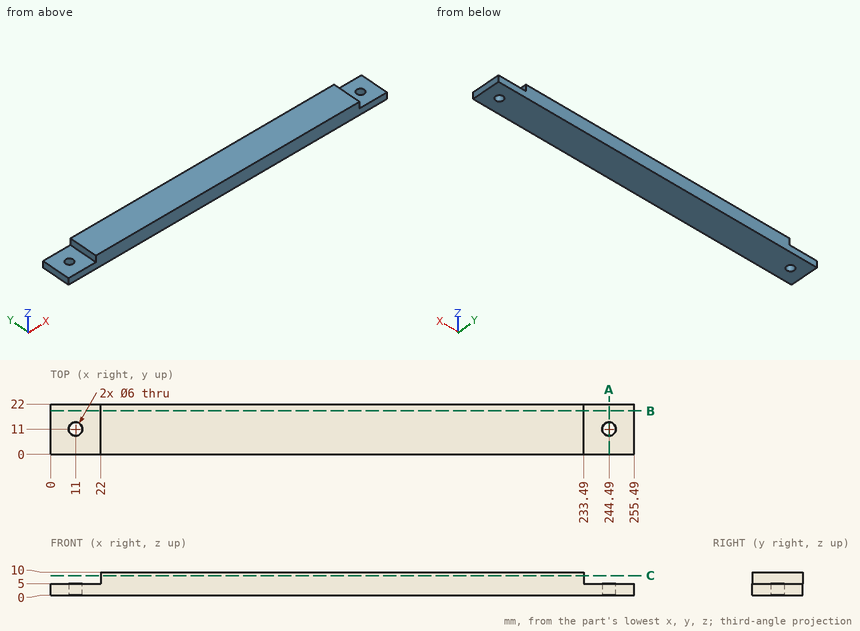
Geometry check sheet. Reference: drawing and pictorial views, mm from the part's lowest x, y, z. Round coordinates to 2 decimals unless told otherwise and drop trailing zeros. Write each loop counter-clockwise with the first axis right and the second up, starting at its lowest first coordinate (ties: lowest second). Pieces come first, ordered by that corner, then holes. Notation, with made-up numbers: (80, 32.5) -> (111, 32.5) arc R13 ccw to (111, 39.5) -> close; hole circle Ø11 at (66, 68). An arc over 180 degrees is marked (long way). Put each result on its own line as item: value.
1) Thickness scan on probe 1 along X at (y, z) = (11, 1.6); probe 2 along Y at (x, z) = (11, 2.7); probe 3 along X at (y, z) = (13.75, 1.5). Record the ranges inside material, lowest first. Write a range as from..to.
Recorded:
probe 1: x = 0..8, 14..241.49, 247.49..255.49
probe 2: y = 0..8, 14..22
probe 3: x = 0..9.8, 12.2..243.29, 245.69..255.49
2) Cross-section at C-C, the plane z = 8.5. Enter the section's corners in (x, y).
Recorded:
outline: (22, 0) -> (233.49, 0) -> (233.49, 22) -> (22, 22) -> close
3) Depth check by flat-ended pin: P1, Ø2.5, axis at y = 7.5, z = 8, coming from the -X side; P2, Ø4, axis at y = 14, z = 8.5, coming from the +X side. Enter the tip coordinate at first touch or a pass-through.
Recorded:
P1: stops at x = 22
P2: stops at x = 233.49
4) Cross-section at A-A, the plane x = 244.49. Enter the section's corners in (y, z).
Recorded:
outline: (0, 0) -> (8, 0) -> (8, 5) -> (0, 5) -> close; (14, 0) -> (22, 0) -> (22, 5) -> (14, 5) -> close
5) Cross-section at B-B, the plane y = 19. Enter the section's corners in (x, z).
Recorded:
outline: (0, 0) -> (255.49, 0) -> (255.49, 5) -> (233.49, 5) -> (233.49, 10) -> (22, 10) -> (22, 5) -> (0, 5) -> close
